The model under review builds one solid part; all positions refer to its coordinate system, in mm. Face numbers are marked on the shaded views. A direction names the side the tool comes from. Coordinates: 2 decimals unless noted, no trailing zeros. Order: outer loops, then holes, each group sorted by start corner. A loop starts at its lowest first (then second) coordinate and runs counter-clockwise, first axis right, second up.
Autodesk Inventor part; units mm, degrees
ref_plane "YZ Plane" through (0, 0, 0) normal (1, 0, 0) x (0, 1, 0)
ref_plane "XZ Plane" through (0, 0, 0) normal (0, 1, 0) x (-1, 0, 0)
ref_plane "XY Plane" through (0, 0, 0) normal (0, 0, 1) x (1, 0, 0)
sketch "スケッチ1" plane through (0, 0, 0) normal (0, 0, 1) x (1, 0, 0)
  circle A0 centre (0, 0) radius 7.5
  dimension "d0" = 15
extrude "押し出し1" add sketch "スケッチ1" along normal blind 3
sketch "スケッチ2" plane through (0, 0, 3) normal (0, 0, 1) x (1, 0, 0)
  line L0 (0, 7.5) -> (6.4952, 3.75)
  line L1 (6.4952, 3.75) -> (6.4952, -3.75)
  line L2 (6.4952, -3.75) -> (0, -7.5)
  line L3 (0, -7.5) -> (-6.4952, -3.75)
  line L4 (-6.4952, -3.75) -> (-6.4952, 3.75)
  line L5 (-6.4952, 3.75) -> (0, 7.5)
  point P0 (0, 0)
  point P1 (0, 0)
  dimension "d8" = 7.5
extrude "押し出し2" add sketch "スケッチ2" along normal blind 5
sketch "スケッチ3" plane through (0, 0, 8) normal (0, 0, 1) x (1, 0, 0)
  circle A0 centre (0, 0) radius 3
  dimension "d5" = 6
extrude "押し出し3" cut sketch "スケッチ3" against normal blind 30
properties part number "頭ねじ" material "アルミニウム"
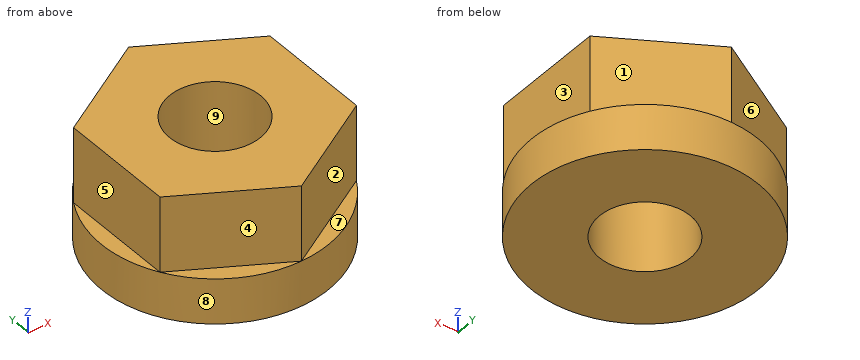
(1) Draft analysis for pull direction X (two halves, no side actions). For the marked faces 6, 7, 8 and 9, state which applies: released by +X, released by -X, zero draft, split by the parting line, or undercut.
A:
face 6: released by -X
face 7: zero draft
face 8: split by the parting line
face 9: undercut
(2) We need section B-B, the plane x = 2.5. Write out the cut boundary in (y, z).
A:
outline: (-7.07, 0) - (-1.66, 0) - (-1.66, 8) - (-6.06, 8) - (-6.06, 3) - (-7.07, 3) - close; (1.66, 0) - (7.07, 0) - (7.07, 3) - (6.06, 3) - (6.06, 8) - (1.66, 8) - close
(3) We need section A-A, the plane y = 0. Write out the cut boundary in (x, z).
A:
outline: (-7.5, 0) - (-3, 0) - (-3, 8) - (-6.5, 8) - (-6.5, 3) - (-7.5, 3) - close; (3, 0) - (7.5, 0) - (7.5, 3) - (6.5, 3) - (6.5, 8) - (3, 8) - close
(4) We need section D-D, the plane y = 5.25. Write out the cut boundary in (x, z).
A:
outline: (-5.36, 0) - (5.36, 0) - (5.36, 3) - (3.9, 3) - (3.9, 8) - (-3.9, 8) - (-3.9, 3) - (-5.36, 3) - close
(5) Wall thickness on probe 1 along Y at (x, z) = (0, 2.5); probe 2 along X at (y, z) = (-3.25, 3.75); probe 3 along Y at (x, z) = (0.25, 7.5): over which ranges is each line inside the solid? List them lowest first.
A:
probe 1: y = -7.5 to -3, 3 to 7.5
probe 2: x = -6.5 to 6.5
probe 3: y = -7.36 to -2.99, 2.99 to 7.36
(6) We need section C-C, the plane z = 2.75. Write out the cut boundary in (x, y), and give its area (3 significant figures).
A:
outline: circle Ø15 at (0, 0); hole circle Ø6 at (0, 0)
area: 148 mm2
(7) For pin 1 Ø4 at (y, z) = (-0.5, 4.5) entering from +X; pin 2 Ø1.5 at (y, z) = (-0.5, 7) entering from +X; pin 3 Ø1.5 at (y, z) = (-1, 6.5) entering from -X; pin 4 Ø4 at (y, z) = (-5.5, 3.5) entering from +X, all flat-tipped, find the tip position at first contact; note any pin that passes through.
A:
pin 1: stops at x = 7.5
pin 2: stops at x = 6.5
pin 3: stops at x = -6.5
pin 4: stops at x = 6.6
(8) Machinability: for the marked faces 1, 2, 3, 4 and 5, which of the approach directions +Z, -Z, +X, -X, +Y, -Y give a long, thin tool a straight path to every point of the face, cutting with its end or side? Answer none if there is none.
A:
face 1: +Z, +X, +Y
face 2: +Z, +X, -Y
face 3: +Z, +X, +Y, -Y
face 4: +Z, -X, -Y
face 5: +Z, -X, +Y, -Y
